Work out the finished part from the listing and answer in its coordinate system (mm). A direction names the side the tool comes from. Give positions to 0.01 mm unless a question says otherwise; leave off trailing zeros. Loops run counter-clockwise (first coordinate to the right, second up) from the corner with the lowest first, then second, coordinate; pieces in that order, holes last. Notation, with made-up numbers: M -34.75,69.5 L -11.75,69.5 A22 ccw -11.75,92.5 Z; hole C -26,-37 d10. An arc over 180 degrees is marked long. Write item = value, one per line. Start each with the question number.
1. For faces 5 (the face through (1, 16, 163.159)), 6 (the face through (38.1, 0, 75)), 7 (the face through (-1, -15.24, 77)), determine the directions among +Z, -Z, +X, -X, +Y, -Y from which every point of the face is accessible in a straight line to the end or side of a thin tool.
2. Consider L1, parallel to Z at x = 5.5, y = 2.5; L2, parallel to Y at x = 21, z = 91; L3, parallel to X at y = 14, z = 193.5. Determine where each line is inside the solid, lowest interval first. Write a range as [from, to].
3. The mould has two halves that part along X. Classify faces 1 (the face through (80.032, 15.88, 192.92)), 2 (the face through (85.9, 15.88, 184.51)), 3 (the face through (-8, 60.96, 162)), 4 (the face through (-38.1, 0, 75)): released by +X, released by -X, zero draft, split by the parting line, or undercut.
4. Section B-B on x = -6 is taken. Determine the outline of the cut face in (y, z), plus the area to 3 significant figures.
5. Section A-A on y = 21.5 is taken. Determine the outline of the cut face in (x, z).
6. Section C-C on y = -6 is taken. Determine the outline of the cut face in (x, z), plus the area to 3 significant figures.
7. Flat-ended cylindrical pins translate along their axes: pin 1 Ø4 at (x, y) = (-63.5, -3) entering from -Z; pin 2 Ø8 at (x, z) = (-38.5, 123.5) entering from +Y; pin 3 Ø5 at (y, z) = (2, 94) entering from -X. Find the tip coordinate at first contact, or state that the pin passes through.
8. Section D-D on z = 115.5 is taken. Determine the outline of the cut face in (x, y).
```python
from build123d import *

# Parameters (mm, degrees)
F0_W     = 76.2
F0_H     = 30.48
F1_DEPTH = 152.4
F3_DEPTH = 76.2
F4_DEPTH = 15.24


with BuildPart() as f1:
    # F0 (on Top) → F1 (new body)
    with BuildSketch(Plane.XY):
        Rectangle(F0_W, F0_H)
    extrude(amount=F1_DEPTH)

    # F2 (on face) → F3 (join)
    with BuildSketch(Plane.XZ.offset(15.24)):
        Polygon((-68.705104, 152.4), (-38.1, 152.4), (38.1, 152.4), (68.705104, 152.4), (103.591479, 217.541933), (95.530655, 221.858859), (64.094205, 163.158833), (0, 163.158833), (-64.094205, 163.158833), (-95.530655, 221.858859), (-103.591479, 217.541933), align=None)
    extrude(amount=-F3_DEPTH)

    # F2 (on face) → F4 (join)
    with BuildSketch(Plane.XZ.offset(15.24)):
        Polygon((-68.705104, 152.4), (-38.1, 152.4), (38.1, 152.4), (68.705104, 152.4), (103.591479, 217.541933), (95.530655, 221.858859), (64.094205, 163.158833), (0, 163.158833), (-64.094205, 163.158833), (-95.530655, 221.858859), (-103.591479, 217.541933), align=None)
    extrude(amount=F4_DEPTH)


solid = f1.part
```
Verdict:
q1.face_5 = +Z, +Y, -Y
q1.face_6 = -Z, +X, +Y, -Y
q1.face_7 = -Z, +X, -X, -Y
q2.L1 = [0, 163.16]
q2.L2 = [-15.24, 15.24]
q2.L3 = [-90.72, -80.34], [80.34, 90.72]
q3.face_1 = undercut
q3.face_2 = released by +X
q3.face_3 = zero draft
q3.face_4 = released by -X
q4.outline = M -30.48,152.4 L -15.24,152.4 L -15.24,0 L 15.24,0 L 15.24,152.4 L 60.96,152.4 L 60.96,163.16 L -30.48,163.16 Z
q4.area = 5,630 mm2
q5.outline = M -103.59,217.54 L -68.71,152.4 L 68.71,152.4 L 103.59,217.54 L 95.53,221.86 L 64.09,163.16 L -64.09,163.16 L -95.53,221.86 Z
q6.outline = M -103.59,217.54 L -68.71,152.4 L -38.1,152.4 L -38.1,0 L 38.1,0 L 38.1,152.4 L 68.71,152.4 L 103.59,217.54 L 95.53,221.86 L 64.09,163.16 L -64.09,163.16 L -95.53,221.86 Z
q6.area = 14,300 mm2
q7.pin_1 = 152.4
q7.pin_2 = 15.24
q7.pin_3 = -38.1
q8.outline = M -38.1,-15.24 L 38.1,-15.24 L 38.1,15.24 L -38.1,15.24 Z
